```python
from build123d import *

# Parameters (mm, degrees)
F1_DEPTH      = 9
F2_R          = 3.99999
F3_R          = 1
F4_R          = 2
F5_W          = 6
F5_H          = 6
F6_DEPTH      = 1
F7_R          = 1.6
F8_DEPTH      = 12.601
F9_R          = 3
F9_R_2        = 1.6
F10_DEPTH     = 2
F12_DEPTH     = 9.001
F13_R         = 3
F14_T1_DEPTH  = 20.400496283
F14_T3_DEPTH  = 8.1624490891
F14_T5_DEPTH  = 15.00002
F14_T7_DEPTH  = 6.3449613941
F14_T9_DEPTH  = 5.5573463904
F14_T11_DEPTH = 4.0573463904
F14_T13_DEPTH = 2.0573563904
F14_T15_DEPTH = 6.7122106995
F14_T18_ANGLE = 90
F14_T20_ANGLE = 135
F14_T22_ANGLE = 90
F14_T24_ANGLE = 90
F14_T26_ANGLE = 90
F14_T28_ANGLE = 45
F14_T30_ANGLE = 90
F14_T32_ANGLE = 135
F14_T34_ANGLE = 90
F14_T36_ANGLE = 45
F14_T38_ANGLE = 90
F14_T40_ANGLE = 90


# Not quite as in the source:
# - a fillet or chamfer that OpenCascade refuses, or shapes differently, is made with other operations: its cross-section is extruded or revolved along the edge and cut away or added
# - a fillet or chamfer is up to 0.001 mm smaller than in the source, because OpenCascade refuses the exact size


with BuildPart() as f1:
    # F0 (on Top) → F1 (new body)
    with BuildSketch(Plane.XY):
        Polygon((0, 4), (0, 0), (12.5766626515, 0), (4.2616702986, -8.3149923529), (8.8578643763, -12.9111864306), (23, 1.2309491931), (23, 13.6), (0, 13.6), (0, 9.6), (19, 9.6), (19, 4), align=None)
    extrude(amount=F1_DEPTH)

    # F2 (radius 4 in the source; OpenCascade refuses exactly that, so slightly less here)
    f2_edges = [f1.edges().sort_by_distance(p)[0] for p in [
        (23, 13.6, 4.5),
        (0, 13.6, 4.5),
        (23, 1.230949, 4.5),
    ]]
    fillet(f2_edges, radius=F2_R)

    # F3
    f3_edges = [f1.edges().sort_by_distance(p)[0] for p in [
        (12.576663, 0, 4.5),
    ]]
    fillet(f3_edges, radius=F3_R)

    # F4
    f4_edges = [f1.edges().sort_by_distance(p)[0] for p in [
        (0, 0, 4.5),
    ]]
    fillet(f4_edges, radius=F4_R)

    # F5 (on face) → F6 (cut)
    with BuildSketch(Plane.XZ):
        with Locations((7.1624490891, 4.5)):
            Rectangle(F5_W, F5_H)
    extrude(amount=-F6_DEPTH, mode=Mode.SUBTRACT)

    # F7 (on face) → F8 (cut, through all)
    with BuildSketch(Plane.XZ.offset(-1)):
        with Locations((7.1624490891, 4.5)):
            Circle(F7_R)
    extrude(amount=-F8_DEPTH, mode=Mode.SUBTRACT)

    # F9 (on face) → F10 (cut)
    with BuildSketch(Plane(origin=(0, 13.6, 0), x_dir=(-1, 0, 0), z_dir=(0, 1, 0))):
        with Locations((-7.1624490891, 4.5)):
            Circle(F9_R)
        with Locations((-7.1624490891, 4.5)):
            Circle(F9_R_2, mode=Mode.SUBTRACT)
    extrude(amount=-F10_DEPTH, mode=Mode.SUBTRACT)

    # F11 (on face) → F12 (cut, through all)
    with BuildSketch(Plane(origin=(0, 0, 0), x_dir=(1, 0, 0), z_dir=(0, 0, -1))):
        Polygon((12.7809664736, 2.6241233026), (14.5487334265, 4.3918902556), (9.9525393488, 8.9880843333), (8.1847723959, 7.2203173803), align=None)
    extrude(amount=-F12_DEPTH, mode=Mode.SUBTRACT)

    # F13
    f13_edges = [f1.edges().sort_by_distance(p)[0] for p in [
        (4.26167, -8.314992, 4.5),
    ]]
    fillet(f13_edges, radius=F13_R)

    # F14: chamfer of 0.8 on 4 edges, made by hand

    # F14_s2 → F14_t1 (cut)
    with BuildSketch(Plane(origin=(-3.4814246111, -3.4814246111, 0), x_dir=(0, 0, 1), z_dir=(0.7071067812, 0.7071067812, 0))):
        Polygon((8.2, 15.3930434455), (9, 14.5930434455), (9, 15.3930434455), align=None)
        Polygon((0, 14.5930434455), (0.8, 15.3930434455), (0, 15.3930434455), align=None)
    extrude(amount=F14_T1_DEPTH, mode=Mode.SUBTRACT)

    # F14_s4 → F14_t3 (cut)
    with BuildSketch(Plane.YZ.offset(2)):
        Polygon((0, 8.2), (0.8, 9), (0, 9), align=None)
        Polygon((0.8, 0), (0, 0.8), (0, 0), align=None)
    extrude(amount=F14_T3_DEPTH, mode=Mode.SUBTRACT)

    # F14_s6 → F14_t5 (cut)
    with BuildSketch(Plane.YZ.offset(3.99999)):
        Polygon((12.8, 0), (13.6, 0.8), (13.6, 0), align=None)
        Polygon((13.6, 8.2), (12.8, 9), (13.6, 9), align=None)
    extrude(amount=F14_T5_DEPTH, mode=Mode.SUBTRACT)

    # F14_s8 → F14_t7 (cut)
    with BuildSketch(Plane(origin=(4.5812245445, 4.5812245445, 0), x_dir=(0, 0, 1), z_dir=(-0.7071067812, -0.7071067812, 0))):
        Polygon((0, -9.6930434455), (0.8, -8.8930434455), (0, -8.8930434455), align=None)
        Polygon((8.2, -8.8930434455), (9, -9.6930434455), (9, -8.8930434455), align=None)
    extrude(amount=F14_T7_DEPTH, mode=Mode.SUBTRACT)

    # F14_s10 → F14_t9 (cut)
    with BuildSketch(Plane(origin=(8.4096516693, -8.4096516693, 0), x_dir=(0, 0, 1), z_dir=(0.7071067812, -0.7071067812, 0))):
        Polygon((0, 2.066131511), (0.8, 2.866131511), (0, 2.866131511), align=None)
        Polygon((8.2, 2.866131511), (9, 2.066131511), (9, 2.866131511), align=None)
    extrude(amount=F14_T9_DEPTH, mode=Mode.SUBTRACT)

    # F14_s12 → F14_t11 (cut)
    with BuildSketch(Plane.XZ.offset(-6.0573463904)):
        Polygon((0.8, 0), (0, 0.8), (0, 0), align=None)
        Polygon((0, 8.2), (0.8, 9), (0, 9), align=None)
    extrude(amount=F14_T11_DEPTH, mode=Mode.SUBTRACT)

    # F14_s14 → F14_t13 (cut)
    with BuildSketch(Plane.XZ.offset(-9.60001)):
        Polygon((0.8, 0), (0, 0.8), (0, 0), align=None)
        Polygon((0, 8.2), (0.8, 9), (0, 9), align=None)
    extrude(amount=F14_T13_DEPTH, mode=Mode.SUBTRACT)

    # F14_s16 → F14_t15 (cut)
    with BuildSketch(Plane.XZ.offset(-9.60001)):
        Polygon((22.2, 0), (23, 0.8), (23, 0), align=None)
        Polygon((23, 8.2), (22.2, 9), (23, 9), align=None)
    extrude(amount=F14_T15_DEPTH, mode=Mode.SUBTRACT)

    # F14_s17 → F14_t18 (revolve, cut)
    with BuildSketch(Plane.YZ.offset(2)):
        Polygon((0.8, 0), (0, 0.8), (0, 0), align=None)
    revolve(axis=Axis((2, 2, 0), (0, 0, -1)), revolution_arc=F14_T18_ANGLE, mode=Mode.SUBTRACT)

    # F14_s19 → F14_t20 (revolve, cut)
    with BuildSketch(Plane(origin=(4.5812245445, 4.5812245445, 0), x_dir=(0, 0, 1), z_dir=(-0.7071067812, -0.7071067812, 0))):
        Polygon((0, -9.6930434455), (0.8, -8.8930434455), (0, -8.8930434455), align=None)
    revolve(axis=Axis((10.1624490891, -1, 0), (0, 0, 1)), revolution_arc=F14_T20_ANGLE, mode=Mode.SUBTRACT)

    # F14_s21 → F14_t22 (revolve, cut)
    with BuildSketch(Plane(origin=(0.0946593164, 0.0946593164, 0), x_dir=(0, 0, 1), z_dir=(0.7071067812, 0.7071067812, 0))):
        Polygon((0, 9.6930434455), (0.8, 8.8930434455), (0, 8.8930434455), align=None)
    revolve(axis=Axis((8.5043109857, -8.3149923529, 0), (0, 0, 1)), revolution_arc=F14_T22_ANGLE, mode=Mode.SUBTRACT)

    # F14_s23 → F14_t24 (revolve, cut)
    with BuildSketch(Plane.XZ.offset(-9.60001)):
        Polygon((22.2, 0), (23, 0.8), (23, 0), align=None)
    revolve(axis=Axis((19.00001, 9.60001, 0), (0, 0, 1)), revolution_arc=F14_T24_ANGLE, mode=Mode.SUBTRACT)

    # F14_s25 → F14_t26 (revolve, cut)
    with BuildSketch(Plane.YZ.offset(3.99999)):
        Polygon((12.8, 0), (13.6, 0.8), (13.6, 0), align=None)
    revolve(axis=Axis((3.99999, 9.60001, 0), (0, 0, 1)), revolution_arc=F14_T26_ANGLE, mode=Mode.SUBTRACT)

    # F14_s27 → F14_t28 (revolve, cut)
    with BuildSketch(Plane(origin=(10.9439046502, 10.9439046502, 0), x_dir=(0, 0, 1), z_dir=(-0.7071067812, -0.7071067812, 0))):
        Polygon((0, -14.5930434455), (0.8, -15.3930434455), (0, -15.3930434455), align=None)
    revolve(axis=Axis((19.00001, 2.8877993005, 0), (0, 0, 1)), revolution_arc=F14_T28_ANGLE, mode=Mode.SUBTRACT)

    # F14_s29 → F14_t30 (revolve, cut)
    with BuildSketch(Plane.YZ.offset(2)):
        Polygon((0, 8.2), (0.8, 9), (0, 9), align=None)
    revolve(axis=Axis((2, 2, 9), (0, 0, -1)), revolution_arc=F14_T30_ANGLE, mode=Mode.SUBTRACT)

    # F14_s31 → F14_t32 (revolve, cut)
    with BuildSketch(Plane(origin=(4.5812245445, 4.5812245445, 0), x_dir=(0, 0, 1), z_dir=(-0.7071067812, -0.7071067812, 0))):
        Polygon((8.2, -8.8930434455), (9, -9.6930434455), (9, -8.8930434455), align=None)
    revolve(axis=Axis((10.1624490891, -1, 9), (0, 0, 1)), revolution_arc=F14_T32_ANGLE, mode=Mode.SUBTRACT)

    # F14_s33 → F14_t34 (revolve, cut)
    with BuildSketch(Plane(origin=(0.0946593164, 0.0946593164, 0), x_dir=(0, 0, 1), z_dir=(0.7071067812, 0.7071067812, 0))):
        Polygon((8.2, 8.8930434455), (9, 9.6930434455), (9, 8.8930434455), align=None)
    revolve(axis=Axis((8.5043109857, -8.3149923529, 9), (0, 0, 1)), revolution_arc=F14_T34_ANGLE, mode=Mode.SUBTRACT)

    # F14_s35 → F14_t36 (revolve, cut)
    with BuildSketch(Plane(origin=(10.9439046502, 10.9439046502, 0), x_dir=(0, 0, 1), z_dir=(-0.7071067812, -0.7071067812, 0))):
        Polygon((8.2, -15.3930434455), (9, -14.5930434455), (9, -15.3930434455), align=None)
    revolve(axis=Axis((19.00001, 2.8877993005, 9), (0, 0, 1)), revolution_arc=F14_T36_ANGLE, mode=Mode.SUBTRACT)

    # F14_s37 → F14_t38 (revolve, cut)
    with BuildSketch(Plane.XZ.offset(-9.60001)):
        Polygon((23, 8.2), (22.2, 9), (23, 9), align=None)
    revolve(axis=Axis((19.00001, 9.60001, 9), (0, 0, 1)), revolution_arc=F14_T38_ANGLE, mode=Mode.SUBTRACT)

    # F14_s39 → F14_t40 (revolve, cut)
    with BuildSketch(Plane.YZ.offset(3.99999)):
        Polygon((13.6, 8.2), (12.8, 9), (13.6, 9), align=None)
    revolve(axis=Axis((3.99999, 9.60001, 9), (0, 0, 1)), revolution_arc=F14_T40_ANGLE, mode=Mode.SUBTRACT)


solid = f1.part
```
Geometry: final body of the model. Coordinates: model frame, mm. A direction names the side the tool comes from. Round coordinates to 2 decimals unless told otherwise and drop trailing zeros. Loops run counter-clockwise (first coordinate to the right, second up) from the corner with the lowest first, then second, coordinate; pieces in that order, holes last.
Item 1: Section B-B, the plane x = 4.5. Output: boundary loops of the cut face in (y, z), plus the area to 3 significant figures.
Checked values:
outline: (0, 0.8) - (0.8, 0) - (4, 0) - (4, 9) - (0.8, 9) - (0, 8.2) - (0, 7.5) - (1, 7.5) - (1, 1.5) - (0, 1.5) - close; (9.6, 0) - (12.8, 0) - (13.6, 0.8) - (13.6, 3.12) - (11.6, 3.12) - (11.6, 5.88) - (13.6, 5.88) - (13.6, 8.2) - (12.8, 9) - (9.6, 9) - close
area: 59.2 mm2
Item 2: Line query: L1, parallel to Y at x = 11.75, z = 4.5; L2, parallel to Y at x = 8, z = 3; L3, parallel to X at y = 11.25, z = 3.25. Output: solid intervals per line, ascending.
Checked values:
L1: y = -10.02 to -7.19, -3.66 to 4, 9.6 to 13.6
L2: y = -12.05 to -4.58, 1 to 4, 9.6 to 11.6
L3: x = 0.36 to 6.16, 8.16 to 22.64
Item 3: Reachability of faces 1 (the flat face through (3, 0, 4)), 2 (the flat face through (8.937, -4.198, 8.594)), 3 (the flat face through (13.652, -3.496, 4.437)) from +Z, -Z, +X, -X, +Y, -Y: full face, straight path, thin tool, end or side. Return the list, or none.
Checked values:
face 1: +Z, -Z, -X
face 2: +Z, -X
face 3: +Z, -Z
Item 4: Section D-D, the plane x = 14. Output: boundary loops of the cut face in (y, z), plus the area to 3 significant figures.
Checked values:
outline: (-7.77, 0.8) - (-6.64, 0) - (-4.94, 0) - (-4.94, 9) - (-6.64, 9) - (-7.77, 8.2) - close; (-3.84, 0) - (4, 0) - (4, 9) - (-3.84, 9) - close; (9.6, 0) - (12.8, 0) - (13.6, 0.8) - (13.6, 8.2) - (12.8, 9) - (9.6, 9) - close
area: 130 mm2
Item 5: Section C-C, the plane y = 5. Output: boundary loops of the cut face in (x, z), plus the area to 3 significant figures.
Checked values:
outline: (19, 0) - (22.2, 0) - (23, 0.8) - (23, 8.2) - (22.2, 9) - (19, 9) - close
area: 35.4 mm2
Item 6: Mould query, pull axis Z, two halves, no side actions, for faces 4 (the flat face through (11.4, 13.2, 8.6)), 5 (the cylindrical face through (7.81, 12.61, 1.57)), 6 (the flat face through (15.25, -6.52, 4.45)), 7 (the flat face through (8.5, 1, 5.9)). Classes: released by +Z, released by -Z, zero draft, split by the parting line, or undercut.
Checked values:
face 4: released by +Z
face 5: undercut
face 6: zero draft
face 7: undercut
Item 7: Section A-A, the plane z = 4.5. State how many separate pieces and enclosed holes the cut face has, plus the area to 3 significant figures.
Checked values:
separate pieces: 3
enclosed holes: 1
area: 244 mm2
Item 8: Contact query for flat-ended pins moving along their axis: P1, Ø0.5, axis at y = 0.5, z = 4.5, coming from the +X side; P2, Ø5, axis at x = 7.16, z = 4.5, coming from the -Y side; P3, Ø2, axis at y = -6, z = 3.5, coming from the +X side; P4, Ø4.5, axis at x = 6.5, z = 5, coming from the +Y side. Output: stop coordinate, or through.
Checked values:
P1: stops at x = 22.38
P2: stops at y = -12.91
P3: stops at x = 16.77
P4: stops at y = 13.6
